Input: part model. Units: mm. Frame: model coordinates. Coordinates: 2 decimals unless noted, no trailing zeros. Order: outer loops, then holes, each group sorted by start corner. A loop starts at its lowest first (then second) coordinate and runs counter-clockwise, first axis right, second up. Notation, with made-up numbers: (29.5, -8.5) - (79.5, -8.5) arc R24 ccw to (79.5, 5.5) - close; hole circle Ø7 at (10, 76.5). An arc over 180 degrees is marked (long way). Use a Markdown table: item, result. Add a question column.
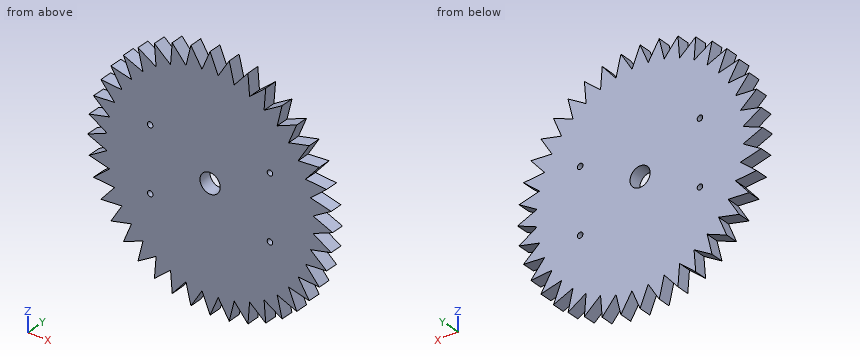
Autodesk Inventor part; units mm, degrees
ref_plane "YZ Plane" through (0, 0, 0) normal (1, 0, 0) x (0, 1, 0)
ref_plane "XZ Plane" through (0, 0, 0) normal (0, 1, 0) x (-1, 0, 0)
ref_plane "XY Plane" through (0, 0, 0) normal (0, 0, 1) x (1, 0, 0)
sketch "Sketch1" plane through (0, 0, 0) normal (0, 1, 0) x (-1, 0, 0)
  circle A0 centre (0, 0) radius 101.6
  dimension "d0" = 203.2
extrude "Extrusion1" add sketch "Sketch1" along normal blind 12.7
sketch "Sketch2" plane through (0, 12.7, 0) normal (0, 1, 0) x (1, 0, 0)
  line L0 (-8.4294, 101.2497) -> (0, 121.6)
  line L1 (0, 121.6) -> (8.4294, 101.2497)
  circle A0 centre (0, 0) radius 101.6
  line L2 (0, 0) -> (0, 122.8461)
  circle A1 centre (0, 0) radius 101.6
  arc A2 (8.4294, 101.2497) -> (-8.4294, 101.2497) centre (0, 0) ccw
  point P0 (0, 101.6)
  dimension "d3" = 45
  dimension "d4" = 20
extrude "Extrusion2" add sketch "Sketch2" against normal up to surface (12.7 mm away) contours L0 L2 A0 | L1 A0 L2
pattern_circular "Circular Pattern1" count 40 over 360 about axis through (0, 0, 0) along (0, 1, 0) of "Extrusion2"
sketch "Sketch3" plane through (0, 12.7, 0) normal (0, 1, 0) x (1, 0, 0)
  circle A0 centre (0, 0) radius 10
  dimension "d10" = 20
extrude "Extrusion3" cut sketch "Sketch3" against normal through all
sketch "Sketch5" plane through (0, 12.7, 0) normal (0, 1, 0) x (1, 0, 0)
  line L0 (-59.436, 31.75) -> (59.436, 31.75)
  line L1 (59.436, 31.75) -> (59.436, -31.75)
  line L2 (59.436, -31.75) -> (-59.436, -31.75)
  line L3 (-59.436, -31.75) -> (-59.436, 31.75)
  circle A0 centre (0, 0) radius 10
  line L4 (-59.436, 31.75) -> (59.436, -31.75) construction
  line L5 (59.436, 31.75) -> (-59.436, -31.75) construction
  dimension "d22" = 63.5
  dimension "d23" = 118.872
hole "Hole1" at (-59.436, 12.7, -31.75) at (-59.436, 12.7, 31.75) at (59.436, 12.7, 31.75) at (59.436, 12.7, -31.75) direction (0, -1, 0) diameter 5.5 end through all
properties part number "BIG ASS GEAR"
1) Cut plane B-B (x = -49). Return the cut outline in (y, z), and give its area (3 significant figures).
2) Cut plane C-C (z = -60). Return the cut outline in (x, y), and give its area (3 significant figures).
3) Contact query for flat-ended pins moving along their axis: P1, Ø1, axis at x = 79.5, y = 5.5, coming from the +Z side; P2, Ø3.5, axis at x = 59.436, z = 31.75, coming from the -Y side; P3, Ø1.5, axis at y = 9.5, z = -1, coming from the -X side; P4, Ø2, axis at y = 10.5, z = 86.5, coming from the -X side. Output: stop coordinate, or through.
4) Material intervals for L1, parallel to Z at x = 0, y = 9; L2, parallel to X at y = 7, z = 89; L3, parallel to Z at x = -96.5, y = 9, sorted ascending.
5) Cut plane A-A (y = 10). State how many separate pieces and enclosed holes the cut face has, and give its area (3 significant figures).
Computed:
| question | item | result |
|---|---|---|
| 1 | outline | (0, -103.05) - (12.7, -103.05) - (12.7, 103.05) - (0, 103.05) - close |
| 1 | area | 2,620 mm2 |
| 2 | outline | (-91.34, 0) - (91.34, 0) - (91.34, 12.7) - (-91.34, 12.7) - close |
| 2 | area | 2,320 mm2 |
| 3 | P1 | stops at z = 83.51 |
| 3 | P2 | passes through |
| 3 | P3 | stops at x = -121 |
| 3 | P4 | stops at x = -85.98 |
| 4 | L1 | z = -121.6 to -10, 10 to 121.6 |
| 4 | L2 | x = -69.22 to -56.17, -53.68 to 53.68, 56.17 to 69.22 |
| 4 | L3 | z = -71.02 to -68.41, -54.27 to -41.33, -39.08 to 39.08, 41.33 to 54.27, 68.41 to 71.02 |
| 5 | separate pieces | 1 |
| 5 | enclosed holes | 5 |
| 5 | area | 38,700 mm2 |
